Source: CAD feature listing. Evaluate the final solid. Frame: model axes, mm. Round coordinates to 2 decimals unless told otherwise and drop trailing zeros. Return JSON: item names as keys, results as strings. Group by question number.
1) Contact query for a flat-ended pin moving along its axis: P1, Ø4, axis at x = 8.5, z = 5, coming from the +Y side. Output: stop coordinate, or through.
2) Mould query, pull axis Z, two halves, no side actions, for faces 1 (the cylindrical face through (17.6, -9.9, 20.5)), 2 (the cylindrical face through (-17.6, -9.9, -20.5)), 3 (the flat face through (35, -10, 0)), 4 (the flat face through (0, -10, -35)). Classes: pulls with the +Z half, pulls with the -Z half, needs draft (parallel to the pull), parting line crosses it, or undercut.
3) Section A-A, the plane y = -6. Give the number of separate pieces and of enclosed holes in the cut face, plus the area to 3 significant figures.
4) Ray query, line 1 (X direction, y = -13.75, z = 19); line 2 (X direction, y = -5.75, z = 8.5); line 3 (X direction, y = -6.5, z = -18). Return the intervals inside material, ascending. Write a range as from..to.
```python
from build123d import *

# Parameters (mm, degrees)
SKETCH2_W           = 70
SKETCH2_H           = 70
BOSS_EXTRUDE1_DEPTH = 20
FILLET1_R           = 1.5
SKETCH3_R           = 2.05
CUT_EXTRUDE1_DEPTH  = 54.385391391


with BuildPart() as part:
    # Sketch2 → Boss-Extrude1 (new body)
    with BuildSketch(Plane(origin=(0, 0, 0), x_dir=(1, 0, 0), z_dir=(0, 1, 0))):
        Rectangle(SKETCH2_W, SKETCH2_H)
    extrude(amount=-BOSS_EXTRUDE1_DEPTH)

    # Sketch1 → Cut-Revolve1 (revolve, cut)
    with BuildSketch(Plane.XY, mode=Mode.PRIVATE) as cut_revolve1_sk:
        with BuildLine():
            Line((0, -17.2), (0, 0))
            Line((0, 0), (21.241684944, 0))
            Line((21.241684944, 0), (21.158851084, -0.511526958))
            add(Edge.make_bspline(
                [(0, -17.2), (0.530678283, -17.2), (1.61157482, -17.183508716), (3.615531125, -17.08588663), (5.944127269, -16.844919371), (8.44843367, -16.370131279), (11.442656399, -15.492934033), (14.579654851, -13.93724298), (17.382164488, -11.402739011), (19.199009229, -8.500896664), (20.23569058, -5.583194157), (20.706490619, -3.313387562), (20.981886079, -1.635929169), (21.096876841, -0.894238762), (21.158851084, -0.511526958)],
                knots=[0, 0, 0, 0, 0.03125, 0.0625, 0.125, 0.1875, 0.25, 0.375, 0.5, 0.625, 0.75, 0.875, 0.9375, 1, 1, 1, 1], degree=3))
        make_face()
    revolve(cut_revolve1_sk.sketch.rotate(Axis((0, -17.2, 0), (0, 1, 0)), 90), axis=Axis((0, -17.2, 0), (0, 1, 0)), mode=Mode.SUBTRACT)

    # Fillet1
    fillet1_edges = [part.edges().sort_by_distance(p)[0] for p in [
        (0, 0, 21.241684944),
    ]]
    fillet(fillet1_edges, radius=FILLET1_R)

    # Sketch3 → Cut-Extrude1 (cut, through all)
    with BuildSketch(Plane(origin=(0, 0, 0), x_dir=(1, 0, 0), z_dir=(0, 1, 0))):
        with Locations(Location((-19, 19, 0), (0, 0, 270))):
            Circle(SKETCH3_R)
        with Locations(Location((19, -19, 0), (0, 0, 90))):
            Circle(SKETCH3_R)
        with Locations(Location((-19, -19, 0), (0, 0, 90))):
            Circle(SKETCH3_R)
        with Locations(Location((19, 19, 0), (0, 0, 270))):
            Circle(SKETCH3_R)
    extrude(amount=-CUT_EXTRUDE1_DEPTH, mode=Mode.SUBTRACT)


solid = part.part
```
Geometry check:
{
 "1": {"P1": "y = -15.21"},
 "2": {"face 1": "undercut", "face 2": "undercut", "face 3": "needs draft", "face 4": "pulls with the -Z half"},
 "3": {"separate pieces": "1", "enclosed holes": "5", "area": "3,590 mm2"},
 "4": {"line 1": "-35..-21.05, -16.95..16.95, 21.05..35", "line 2": "-35..-18.23, 18.23..35", "line 3": "-35..-20.79, -17.21..-8.45, 8.45..17.21, 20.79..35"}
}
